Autodesk Inventor part; units mm, degrees
ref_plane "YZ Plane" through (0, 0, 0) normal (1, 0, 0) x (0, 1, 0)
ref_plane "XZ Plane" through (0, 0, 0) normal (0, 1, 0) x (-1, 0, 0)
ref_plane "XY Plane" through (0, 0, 0) normal (0, 0, 1) x (1, 0, 0)
sketch "Sketch1" plane through (0, 0, 0) normal (0, 1, 0) x (-1, 0, 0)
  line L0 (-17.8956, 13.1221) -> (-17.8956, -9.4779)
  line L1 (-17.8956, -9.4779) -> (-5.5956, -9.4779)
  line L2 (-5.5956, -9.4779) -> (-5.5956, 13.1221)
  line L3 (-5.5956, 13.1221) -> (-17.8956, 13.1221)
  point P0 (0, 0)
  dimension "d0" = 22.6
  dimension "d1" = 12.3
extrude "Extrusion1" add sketch "Sketch1" along normal blind 23.5
sketch "Sketch2" plane through (17.8956, 0, -9.4779) normal (0, 0, -1) x (-1, 0, 0)
  line L0 (0, 0) -> (0, 23.5)
  line L1 (12.3, 0) -> (12.3, 23.5)
  line L2 (0, 17.2) -> (12.3, 17.2)
  line L3 (12.3, 17.2) -> (12.3, 19.5)
  line L4 (12.3, 19.5) -> (0, 19.5)
  line L5 (0, 19.5) -> (0, 17.2)
  line L6 (0, 0) -> (12.3, 0)
  point P0 (17.8956, 0)
  point P1 (0, 19.5)
  dimension "d4" = 17.2
  dimension "d5" = 2.3
extrude "Extrusion2" add sketch "Sketch2" along normal blind 5 contours L0 L4 L1 L2
sketch "Sketch3" plane through (5.5956, 0, 13.1221) normal (0, 0, 1) x (1, 0, 0)
  line L0 (0, 19.5) -> (12.3, 19.5)
  line L1 (12.3, 17.2) -> (0, 17.2)
  line L2 (12.3, 19.5) -> (0, 19.5)
  line L3 (0, 19.5) -> (0, 17.2)
  line L4 (0, 17.2) -> (12.3, 17.2)
  line L5 (12.3, 17.2) -> (12.3, 19.5)
  point P0 (-5.5956, 0)
  point P1 (0, 19.5)
  point P2 (12.3, 17.2)
extrude "Extrusion3" add sketch "Sketch3" along normal blind 5
sketch "Sketch4" plane through (0, 23.5, 0) normal (0, 1, 0) x (1, 0, 0)
  circle A0 centre (11.7456, 3.4779) radius 2.35
  line L0 (17.8956, 9.4779) -> (5.5956, 9.4779)
  point P0 (0, 0)
  dimension "d10" = 4.7
  dimension "d11" = 6
extrude "Extrusion4" add sketch "Sketch4" along normal blind 4.5
properties part number "testingservo"
Can you work these out from the model? Positions are in its coordinate system, mm. A direction names the side the tool comes from. Coordinates: 2 decimals unless noted, no trailing zeros. Write each loop counter-clockwise with the first axis right and the second up, starting at its lowest first coordinate (ties: lowest second). Pieces come first, ordered by that corner, then holes. Notation, with made-up numbers: (79.5, 69) - (107.5, 69) arc R27 ccw to (107.5, 102) - close; hole circle Ø8 at (59, 66). An arc over 180 degrees is marked (long way). Return JSON: item names as keys, results as strings. Group by question number.
Item 1: Please list where these lines run through material, in increasing order: probe 1 along Y at (x, z) = (14.5, -1); probe 2 along Y at (x, z) = (11.25, -10); probe 3 along Z at (x, y) = (8.5, 6.5).
Item 2: If we section it at A-A (x = 14.5): Write out the boundary of the cut face in (y, z).
Item 3: If we section it at B-B (z = -2.5): Write out the boundary of the cut face in (x, y).
Item 4: Which directions (+Z, -Z, +X, -X, +Y, -Y) give clear straight access to the entire face, cutting with the end or side of a thin tool? Please do faces 1 (the face through (12, 19.5, -12)), 2 (the face through (9.4, 25.72, -3.37)), 3 (the face through (12, 8, 13.122)), 4 (the face through (12, 17.2, -12)), 5 (the face through (12, 21, 13.122)).
Item 5: I'm going to push flat-ended pins straight in: pin 1 Ø6 at (x, y) = (9, 6.5) entering from -Z; pin 2 Ø1.5 at (x, y) = (15.5, 9) entering from +Z; pin 3 Ø4 at (x, z) = (10, 16.5) entering from +Y. Where does each tip first touch, or does it pass through?
Item 6: If we section it at D-D (x = 10.5): Write out the boundary of the cut face in (y, z).
Item 7: If we section it at C-C (y = 7): Write out the boundary of the cut face in (x, z).
Return value:
{
 "1": {"probe 1": "y = 0 to 23.5", "probe 2": "y = 17.2 to 19.5", "probe 3": "z = -9.48 to 13.12"},
 "2": {"outline": "(0, -9.48) - (17.2, -9.48) - (17.2, -14.48) - (19.5, -14.48) - (19.5, -9.48) - (23.5, -9.48) - (23.5, 13.12) - (19.5, 13.12) - (19.5, 18.12) - (17.2, 18.12) - (17.2, 13.12) - (0, 13.12) - close"},
 "3": {"outline": "(5.6, 0) - (17.9, 0) - (17.9, 23.5) - (13.88, 23.5) - (13.88, 28) - (9.61, 28) - (9.61, 23.5) - (5.6, 23.5) - close"},
 "4": {"face 1": "-Z, +X, -X, +Y", "face 2": "+Y", "face 3": "+Z, +X, -X, -Y", "face 4": "-Z, +X, -X, -Y", "face 5": "+Z, +X, -X, +Y"},
 "5": {"pin 1": "stops at z = -9.48", "pin 2": "stops at z = 13.12", "pin 3": "stops at y = 19.5"},
 "6": {"outline": "(0, -9.48) - (17.2, -9.48) - (17.2, -14.48) - (19.5, -14.48) - (19.5, -9.48) - (23.5, -9.48) - (23.5, -5.47) - (28, -5.47) - (28, -1.49) - (23.5, -1.49) - (23.5, 13.12) - (19.5, 13.12) - (19.5, 18.12) - (17.2, 18.12) - (17.2, 13.12) - (0, 13.12) - close"},
 "7": {"outline": "(5.6, -9.48) - (17.9, -9.48) - (17.9, 13.12) - (5.6, 13.12) - close"}
}
